Source: three-view drawing plus pictorial views. Frame: mm from the lowest corner of the part. A direction names the side the tool comes from. Round coordinates to 2 decimals unless told otherwise and drop trailing zeros. Order: outer loops, then holes, each group sorted by start corner. A loop starts at its lowest first (then second) coordinate and runs counter-clockwise, first axis right, second up. Notation, with made-up numbers: (58, 43.25) -> (110, 43.25) arc R17 cw to (110, 56.25) -> close; hole circle Ø6 at (-26, 19.25). An arc over 180 degrees is marked (long way). Answer as CSV lines item,"result".
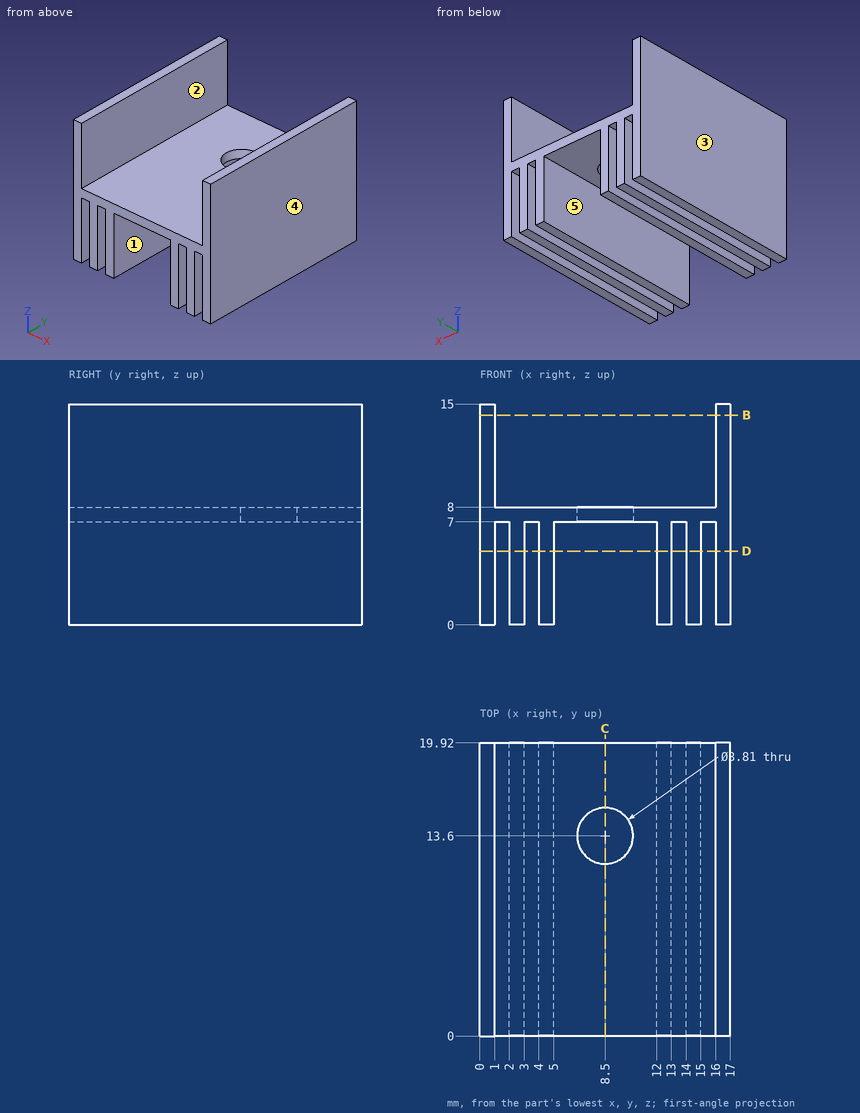
1. Section query B-B on z = 14.25. Return loops of the section in (x, y).
Results below:
outline,"(0, 0) -> (1, 0) -> (1, 19.92) -> (0, 19.92) -> close; (16, 0) -> (17, 0) -> (17, 19.92) -> (16, 19.92) -> close"
2. Mould query, pull axis X, two halves, no side actions, for the marked faces 3, 4 and 5. Classes: released by +X, released by -X, zero draft, split by the parting line, or undercut.
Results below:
face 3,"released by -X"
face 4,"released by +X"
face 5,"undercut"
3. Pin query (flat end, axial travel): pin 1 (0.8 mm diameter, centred on x = 1.5, y = 6.5, fed in from -Z); pin 2 (7.5 mm diameter, centred on x = 9, y = 13, fed in from -Z); pin 3 (1.5 mm diameter, centred on x = 14.5, y = 2, fed in from +Z). Return the tip coordinate at first contact, or that it passes through.
Results below:
pin 1,"z = 7"
pin 2,"z = 0"
pin 3,"z = 8"
4. Section query C-C on x = 8.5. Return loops of the section in (y, z) (1 decimal), and give its area (3 significant figures).
Results below:
outline,"(0, 7) -> (11.7, 7) -> (11.7, 8) -> (0, 8) -> close; (15.5, 7) -> (19.9, 7) -> (19.9, 8) -> (15.5, 8) -> close"
area,"16.1 mm2"
5. Line query: L1, parallel to X at y = 5.25, z = 6.75; L2, parallel to Y at x = 8.5, z = 7.6 (1 decimal); L3, parallel to X at y = 11.25, z = 10.25. Output: solid intervals per line, ascending. Write a range as [from, to].
Results below:
L1,"[0, 1], [2, 3], [4, 5], [12, 13], [14, 15], [16, 17]"
L2,"[0, 11.7], [15.5, 19.9]"
L3,"[0, 1], [16, 17]"
6. Section query D-D on z = 5. Return loops of the section in (x, y).
Results below:
outline,"(0, 0) -> (1, 0) -> (1, 19.92) -> (0, 19.92) -> close; (2, 0) -> (3, 0) -> (3, 19.92) -> (2, 19.92) -> close; (4, 0) -> (5, 0) -> (5, 19.92) -> (4, 19.92) -> close; (12, 0) -> (13, 0) -> (13, 19.92) -> (12, 19.92) -> close; (14, 0) -> (15, 0) -> (15, 19.92) -> (14, 19.92) -> close; (16, 0) -> (17, 0) -> (17, 19.92) -> (16, 19.92) -> close"
7. Reachability of the marked faces 1 and 2 from +Z, -Z, +X, -X, +Y, -Y: full face, straight path, thin tool, end or side. Return the list, or none.
Results below:
face 1,"-Z, +Y, -Y"
face 2,"+Z, +Y, -Y"
